Read the model definition and answer for the solid it produces. Units are mm, in the model's axes. A direction names the side the tool comes from. Coordinates: 2 decimals unless noted, no trailing zeros. Loops run counter-clockwise (first coordinate to the right, second up) from the corner with the lowest first, then second, coordinate; pieces in that order, holes last.
from build123d import *

# Parameters (mm, degrees)
CROQUIS1_R              = 35
SALIENTE_EXTRUIR1_DEPTH = 8
CROQUIS2_R              = 2.35
CORTAR_EXTRUIR1_DEPTH   = 5


with BuildPart() as part:
    # Croquis1 → Saliente-Extruir1 (new body)
    with BuildSketch(Plane.XY):
        Circle(CROQUIS1_R)
        with BuildLine():
            Line((2.90473751, 2.75), (2.90473751, -2.75))
            ThreePointArc((2.90473751, -2.75), (-4, 0), (2.90473751, 2.75))
        make_face(mode=Mode.SUBTRACT)
    extrude(amount=SALIENTE_EXTRUIR1_DEPTH)

    # Croquis2 → Cortar-Extruir1 (cut)
    with BuildSketch(Plane.XY.offset(8)):
        with Locations((27, 0)):
            Circle(CROQUIS2_R)
        with Locations((13.5, -23.382685902)):
            Circle(CROQUIS2_R)
        with Locations((-13.5, -23.382685902)):
            Circle(CROQUIS2_R)
        with Locations((-27, 0)):
            Circle(CROQUIS2_R)
        with Locations((-13.5, 23.382685902)):
            Circle(CROQUIS2_R)
        with Locations((13.5, 23.382685902)):
            Circle(CROQUIS2_R)
    extrude(amount=-CORTAR_EXTRUIR1_DEPTH, mode=Mode.SUBTRACT)


solid = part.part
Item 1: A cutting plane is placed at B-B on x = 0. Determine the outline of the cut face in (y, z), then the cut area to 3 significant figures.
Numbers:
outline: (-35, 0) - (-4, 0) - (-4, 8) - (-35, 8) - close; (4, 0) - (35, 0) - (35, 8) - (4, 8) - close
area: 496 mm2
Item 2: A cutting plane is placed at A-A on y = 0. Determine the outline of the cut face in (x, z).
Numbers:
outline: (-35, 0) - (-4, 0) - (-4, 8) - (-24.65, 8) - (-24.65, 3) - (-29.35, 3) - (-29.35, 8) - (-35, 8) - close; (2.9, 0) - (35, 0) - (35, 8) - (29.35, 8) - (29.35, 3) - (24.65, 3) - (24.65, 8) - (2.9, 8) - close
Item 3: Find the intervals of material crossed by line 1 along X through (y, z) = (-22.5, 5.5); line 2 along X through (y, z) = (-25, 3.5); line 3 along Y through (x, z) = (13.5, 4.5), in increasing order.
Numbers:
line 1: x = -26.81 to -15.68, -11.32 to 11.32, 15.68 to 26.81
line 2: x = -24.49 to -15.2, -11.8 to 11.8, 15.2 to 24.49
line 3: y = -32.29 to -25.73, -21.03 to 21.03, 25.73 to 32.29
Item 4: A cutting plane is placed at C-C on z = 4.75. Determine the outline of the cut face in (x, y), then the cut area to 3 significant figures.
Numbers:
outline: circle Ø70 at (0, 0); hole circle Ø4.7 at (-27, 0); hole circle Ø4.7 at (-13.5, -23.38); hole circle Ø4.7 at (-13.5, 23.38); hole (2.9, -2.75) - (2.9, 2.75) arc R4 ccw (long way) to start; hole circle Ø4.7 at (13.5, -23.38); hole circle Ø4.7 at (13.5, 23.38); hole circle Ø4.7 at (27, 0)
area: 3,700 mm2
Item 5: Determine the mould class of faces 1 (the face through (-28, -21, 4)), 2 (the face through (24.652, 0.103, 5.535)), 3 (the face through (0, -7, 0)) for opening direction X: released by +X, released by -X, zero draft, split by the parting line, or undercut.
Numbers:
face 1: split by the parting line
face 2: undercut
face 3: zero draft
Item 6: Given pin 1 (1.4 mm diameter, centred on x = -26, y = 1, fed in from +Z); pin 2 (3 mm diameter, centred on x = 13, z = 1.5, fed in from -Y); pin 3 (4 mm diameter, centred on x = 3.5, z = 6.5, fed in from +Y), each flat-ended and moving along its own axis, determine where each tip first touches the part or whether it passes through.
Numbers:
pin 1: stops at z = 3
pin 2: stops at y = -33.06
pin 3: stops at y = 34.97
Item 7: A cutting plane is placed at D-D on x = 27. Determine the outline of the cut face in (y, z), then the cut area to 3 significant figures.
Numbers:
outline: (-22.27, 0) - (22.27, 0) - (22.27, 8) - (2.35, 8) - (2.35, 3) - (-2.35, 3) - (-2.35, 8) - (-22.27, 8) - close
area: 333 mm2
Item 8: Which of the six approach directions +Z, -Z, +X, -X, +Y, -Y give full straight-line access (tool end or side, diameter ignored) to faces 4 (the face through (2.905, 0, 4)), 5 (the face through (0, -7, 8)), 6 (the face through (-27, 0, 3))?
Numbers:
face 4: +Z, -Z
face 5: +Z, +X, -X, +Y, -Y
face 6: +Z
